Autodesk Fusion 360 part; units mm, degrees
sketch "Sketch1" plane through (0, 0, 0) normal (1, 0, 0) x (0, 1, 0)
  circle A0 centre (0, 0) radius 0.5
  line L0 (0.325, -0.325) -> (-0.325, -0.325)
  line L1 (-0.325, -0.325) -> (-0.325, 0.325)
  line L2 (-0.325, 0.325) -> (0.325, 0.325)
  line L3 (0.325, 0.325) -> (0.325, -0.325)
  line L4 (0.325, -0.325) -> (-0.325, 0.325) construction
  line L5 (-0.325, -0.325) -> (0.325, 0.325) construction
  dimension "d1" = 1
  dimension "d2" = 0.65
  dimension "d3" = 0.65
extrude "Extrude1" add sketch "Sketch1" along normal blind 20 contours A0 | L0 L1 L2 L3
sketch "Sketch2" plane through (20, 0, 0) normal (1, 0, 0) x (0, 1, 0)
  circle A0 centre (0, 0) radius 0.5
  line L0 (0.325, -0.325) -> (-0.325, -0.325)
  line L1 (-0.325, -0.325) -> (-0.325, 0.325)
  line L2 (-0.325, 0.325) -> (0.325, 0.325)
  line L3 (0.325, 0.325) -> (0.325, -0.325)
  line L4 (0.325, -0.325) -> (-0.325, 0.325) construction
  line L5 (-0.325, -0.325) -> (0.325, 0.325) construction
  dimension "d8" = 0.65
  dimension "d9" = 0.65
extrude "Extrude2" add sketch "Sketch2" along normal blind 1.755 contours L0 L1 L2 L3
extrude "Extrude3" add sketch "Sketch1" against normal blind 1.755 contours L0 L1 L2 L3
sketch "Sketch3" plane through (0, 0, -0.325) normal (0, 0, -1) x (1, 0, 0)
  line L0 (20, 0.325) -> (20, -0.325)
  line L1 (20, -0.325) -> (21.755, -0.325)
  line L2 (21.755, -0.325) -> (21.755, 0.325)
  line L3 (21.755, 0.325) -> (20, 0.325)
  line L4 (21.755, 0.325) -> (21.105, 0.325)
  line L5 (21.105, 0.325) -> (21.105, -0.325)
  line L6 (21.105, -0.325) -> (21.755, -0.325)
  line L7 (21.755, -0.325) -> (21.755, 0.325)
  line L8 (21.755, 0.325) -> (21.105, -0.325) construction
  line L9 (21.105, 0.325) -> (21.755, -0.325) construction
  point P0 (21.43, 0)
  dimension "d14" = 0.65
  dimension "d15" = 0.65
sketch "Sketch4" plane through (0, 0, -0.325) normal (0, 0, -1) x (1, 0, 0)
  line L0 (0, -0.325) -> (0, 0.325)
  line L1 (0, 0.325) -> (-1.755, 0.325)
  line L2 (-1.755, 0.325) -> (-1.755, -0.325)
  line L3 (-1.755, -0.325) -> (0, -0.325)
  line L4 (-1.105, -0.325) -> (-1.755, -0.325)
  line L5 (-1.755, -0.325) -> (-1.755, 0.325)
  line L6 (-1.755, 0.325) -> (-1.105, 0.325)
  line L7 (-1.105, 0.325) -> (-1.105, -0.325)
  line L8 (-1.105, -0.325) -> (-1.755, 0.325) construction
  line L9 (-1.755, -0.325) -> (-1.105, 0.325) construction
  point P0 (-1.43, 0)
  dimension "d17" = 0.65
  dimension "d18" = 0.65
extrude "Extrude4" add sketch "Sketch4" sketch "Sketch3" along normal blind 2.75 contours L1 L2 L3 L4 L5 L6 L7 of sketch 2 contours L1 L2 L3 L4 L5 L6 L7
fillet "Fillet1" radius 0.5 2 edges at (-1.105, 0, -0.325) (21.105, 0, -0.325)
fillet "Fillet2" radius 1 2 edges at (-1.755, 0, 0.325) (21.755, 0, 0.325)
fillet "Fillet3" radius 0.2 28 edges at (-1.43, -0.325, -3.075) (-1.105, 0, -3.075) (-1.43, 0.325, -3.075) (-1.755, 0, -3.075) (-0.9586, -0.325, -0.4714) (-1.105, -0.325, -1.95) (-0.3775, -0.325, 0.325) (-1.4621, -0.325, 0.0321) (-1.755, -0.325, -1.875) (-0.3775, 0.325, 0.325) (-1.4621, 0.325, 0.0321) (-1.755, 0.325, -1.875) (-0.9586, 0.325, -0.4714) (-1.105, 0.325, -1.95) (20.3775, -0.325, 0.325) (21.4621, -0.325, 0.0321) (21.755, -0.325, -1.875) (21.105, -0.325, -1.95) (20.9586, -0.325, -0.4714) (21.755, 0.325, -1.875) (21.4621, 0.325, 0.0321) (20.3775, 0.325, 0.325) (20.9586, 0.325, -0.4714) (21.105, 0.325, -1.95) (21.43, 0.325, -3.075) (21.755, 0, -3.075) (21.43, -0.325, -3.075) (21.105, 0, -3.075)
equation "d1 = width"
equation "d2 = d3"
equation "d3 = d1 * 0.65"
equation "width = 1 mm"
equation "baseLenght = 20 mm"
equation "d6 = baseLenght"
equation "d8 = width * 0.65"
equation "d9 = d8"
equation "d14 = width * 0.65"
equation "d15 = d14"
equation "d17 = width * 0.65"
equation "d18 = d17"
equation "d26 = 0.2 * width"
The listing builds one solid part. Answer for the finished solid, in the listing's coordinates (mm). Give positions to 0.01 mm unless a question says otherwise; leave off trailing zeros. Order: outer loops, then holes, each group sorted by start corner. A loop starts at its lowest first (then second) coordinate and runs counter-clockwise, first axis right, second up. Notation, with made-up numbers: (5.25, -24.75) -> (58.25, -24.75) arc R24 ccw to (58.25, -7.75) -> close; hole circle Ø6 at (14.25, 79.5). An arc over 180 degrees is marked (long way). Answer as CSV lines item,"result". Start each with the question number.
Q1. Given pin 1 (1.2 mm diameter, centred on x = 21, z = -1, fed in from -Y) (3 decimals); pin 2 (1.2 mm diameter, centred on x = 21, z = -1.5, fed in from +Y) (3 decimals); pin 3 (0.5 mm diameter, centred on y = 0, z = 0, fed in from +X), each flat-ended and moving along its own axis, determine where each tip first touches the part or whether it passes through.
Q2. A cutting plane is placed at B-B (x = 10.75). Determine the outline of the cut face in (y, z), then the cut area to 3 significant figures.
Q3. A cutting plane is placed at A-A (z = -2.5). Determine the outline of the cut face in (x, y) (3 decimals), then the cut area to 3 significant figures.
Q4. Find the intervals of material crossed by L1, parallel to X at y = 0.1, z = -1.95 (3 decimals); L2, parallel to X at y = 0.25, z = -2.7; L3, parallel to X at y = -0.4, z = 0.05, in increasing order.
Results found:
1,pin 1,"y = -0.325"
1,pin 2,"y = 0.325"
1,pin 3,"x = 21.66"
2,outline,"circle Ø1 at (0, 0)"
2,area,"0.785 mm2"
3,outline,"(-1.755, -0.125) arc R0.2 ccw to (-1.555, -0.325) -> (-1.305, -0.325) arc R0.2 ccw to (-1.105, -0.125) -> (-1.105, 0.125) arc R0.2 ccw to (-1.305, 0.325) -> (-1.555, 0.325) arc R0.2 ccw to (-1.755, 0.125) -> close; (21.105, -0.125) arc R0.2 ccw to (21.305, -0.325) -> (21.555, -0.325) arc R0.2 ccw to (21.755, -0.125) -> (21.755, 0.125) arc R0.2 ccw to (21.555, 0.325) -> (21.305, 0.325) arc R0.2 ccw to (21.105, 0.125) -> close"
3,area,"0.776 mm2"
4,L1,"-1.755 to -1.105, 21.105 to 21.755"
4,L2,"-1.71 to -1.15, 21.15 to 21.71"
4,L3,"0 to 20"
